```python
from build123d import *

# Parameters (mm, degrees)
SKETCH1_R           = 1.168758958
BOSS_EXTRUDE1_DEPTH = 3


with BuildPart() as part:
    # Sketch1 → Boss-Extrude1 (new body)
    # profile 1 of 4: a face of its own
    with BuildSketch(Plane.XY):
        Polygon((26.025, 45.5), (23.35, 45.5), (23.35, -45.5), (26.025, -45.5), (26.025, -40.5), (32.025, -40.5), (32.025, -45.5), (61.375, -45.5), (61.375, -40.5), (67.375, -40.5), (67.375, -45.5), (70.05, -45.5), (70.05, 45.5), (67.375, 45.5), (67.375, 40.5), (61.375, 40.5), (61.375, 45.5), (32.025, 45.5), (32.025, 40.5), (26.025, 40.5), align=None)
        with Locations((29.025, -37.05)):
            Circle(SKETCH1_R, mode=Mode.SUBTRACT)
        with Locations((64.375, -37.05)):
            Circle(SKETCH1_R, mode=Mode.SUBTRACT)
        with Locations((29.025, 37.05)):
            Circle(SKETCH1_R, mode=Mode.SUBTRACT)
        with Locations((64.375, 37.05)):
            Circle(SKETCH1_R, mode=Mode.SUBTRACT)
    # profile 2 of 4: a face of its own
    with BuildSketch(Plane.XY):
        Polygon((-20.675, 45.5), (-23.35, 45.5), (-23.35, -45.5), (-20.675, -45.5), (-20.675, -40.5), (-14.675, -40.5), (-14.675, -45.5), (14.675, -45.5), (14.675, -40.5), (20.675, -40.5), (20.675, -45.5), (23.35, -45.5), (23.35, 45.5), (20.675, 45.5), (20.675, 40.5), (14.675, 40.5), (14.675, 45.5), (-14.675, 45.5), (-14.675, 40.5), (-20.675, 40.5), align=None)
        with Locations((-17.675, -37.05)):
            Circle(SKETCH1_R, mode=Mode.SUBTRACT)
        with Locations((17.675, -37.05)):
            Circle(SKETCH1_R, mode=Mode.SUBTRACT)
        with Locations((-17.675, 37.05)):
            Circle(SKETCH1_R, mode=Mode.SUBTRACT)
        with Locations((17.675, 37.05)):
            Circle(SKETCH1_R, mode=Mode.SUBTRACT)
    # profile 3 of 4: a face of its own
    with BuildSketch(Plane.XY):
        Polygon((72.725, 45.5), (70.05, 45.5), (70.05, -45.5), (72.725, -45.5), (72.725, -40.5), (78.725, -40.5), (78.725, -45.5), (108.075, -45.5), (108.075, -40.5), (114.075, -40.5), (114.075, -45.5), (116.75, -45.5), (116.75, 45.5), (114.075, 45.5), (114.075, 40.5), (108.075, 40.5), (108.075, 45.5), (78.725, 45.5), (78.725, 40.5), (72.725, 40.5), align=None)
        with Locations((75.725, -37.05)):
            Circle(SKETCH1_R, mode=Mode.SUBTRACT)
        with Locations((111.075, -37.05)):
            Circle(SKETCH1_R, mode=Mode.SUBTRACT)
        with Locations((75.725, 37.05)):
            Circle(SKETCH1_R, mode=Mode.SUBTRACT)
        with Locations((111.075, 37.05)):
            Circle(SKETCH1_R, mode=Mode.SUBTRACT)
    # profile 4 of 4: a face of its own
    with BuildSketch(Plane.XY):
        Polygon((119.425, 45.5), (116.75, 45.5), (116.75, -45.5), (119.425, -45.5), (119.425, -40.5), (125.425, -40.5), (125.425, -45.5), (154.775, -45.5), (154.775, -40.5), (160.775, -40.5), (160.775, -45.5), (163.45, -45.5), (163.45, 45.5), (160.775, 45.5), (160.775, 40.5), (154.775, 40.5), (154.775, 45.5), (125.425, 45.5), (125.425, 40.5), (119.425, 40.5), align=None)
        with Locations((122.425, -37.05)):
            Circle(SKETCH1_R, mode=Mode.SUBTRACT)
        with Locations((157.775, -37.05)):
            Circle(SKETCH1_R, mode=Mode.SUBTRACT)
        with Locations((122.425, 37.05)):
            Circle(SKETCH1_R, mode=Mode.SUBTRACT)
        with Locations((157.775, 37.05)):
            Circle(SKETCH1_R, mode=Mode.SUBTRACT)
    extrude(amount=BOSS_EXTRUDE1_DEPTH)


solid = part.part
```
Could you check a few things on this model? Use its own coordinates, in mm. Coordinates: 2 decimals unless noted, no trailing zeros. Put each result on its own line as item: value. Start each with the question number.
(1) I need wall thicknesses on line 1 (Y direction, x = 65, z = 2.7); line 2 (Y direction, x = 19.5, z = 0.5). Which ranges of each line are inside material? Lowest first, please. Write a range as from..to.
(2) Suppose I cut it at A-A on z = 1.55. Count the separate pieces of the cut face and the enclosed holes in it, then the cut area to 3 significant figures.
(3) Will this pin go through, and if not, where does the flat tip stop? P1, Ø0.9, axis at x = 18, z = 1.5, coming from the +Y side.
Solutions:
1. line 1: y = -40.5..-38.04, -36.06..36.06, 38.04..40.5
1. line 2: y = -40.5..40.5
2. separate pieces: 1
2. enclosed holes: 16
2. area: 16,500 mm2
3. P1: stops at y = 40.5
